Design review of the part built by this model. Coordinates are the model's own, in mm. A direction names the side the tool comes from. Coordinates: 2 decimals unless noted, no trailing zeros. Order: outer loops, then holes, each group sorted by start corner. A loop starts at its lowest first (then second) coordinate and runs counter-clockwise, first axis right, second up. Notation, with made-up numbers: M 54.25,-2.75 L 66.25,-2.75 A32 cw 66.25,28.25 Z; hole C 16.5,52 d10. An arc over 180 degrees is marked long. Answer in a Markdown table with one row per item.
from build123d import *

# Parameters (mm, degrees)
F0_R     = 76.2
F1_DEPTH = 6.35
F3_DEPTH = 3.81


with BuildPart() as f1:
    # F0 (on Top) → F1 (new body)
    with BuildSketch(Plane.XY):
        Circle(F0_R)
    extrude(amount=F1_DEPTH)

    # F2 (on face) → F3 (cut)
    with BuildSketch(Plane.XY.offset(6.35)):
        with BuildLine():
            Line((0, 76.2), (-1.27, 76.2))
            Line((-1.27, 76.2), (-1.27, 76.1894159316))
            ThreePointArc((-1.27, 76.1894159316), (-0.6350220513, 76.197353937), (0, 76.2))
        make_face()
        with BuildLine():
            Line((1.27, 76.2), (0, 76.2))
            ThreePointArc((0, 76.2), (0.6350220513, 76.197353937), (1.27, 76.1894159316))
            Line((1.27, 76.1894159316), (1.27, 76.2))
        make_face()
        with BuildLine():
            ThreePointArc((0, -76.2), (-0.6350220513, -76.197353937), (-1.27, -76.1894159316))
            Line((-1.27, -76.1894159316), (-1.27, -76.2))
            Line((-1.27, -76.2), (0, -76.2))
        make_face()
        with BuildLine():
            Line((1.27, -76.2), (1.27, -76.1894159316))
            ThreePointArc((1.27, -76.1894159316), (0.6350220513, -76.197353937), (0, -76.2))
            Line((0, -76.2), (1.27, -76.2))
        make_face()
        with BuildLine():
            ThreePointArc((1.27, 76.1894159316), (0.6350220513, 76.197353937), (0, 76.2))
            ThreePointArc((0, 76.2), (-0.6350220513, 76.197353937), (-1.27, 76.1894159316))
            Line((-1.27, 76.1894159316), (-1.27, -76.1894159316))
            ThreePointArc((-1.27, -76.1894159316), (-0.6350220513, -76.197353937), (0, -76.2))
            ThreePointArc((0, -76.2), (0.6350220513, -76.197353937), (1.27, -76.1894159316))
            Line((1.27, -76.1894159316), (1.27, 76.1894159316))
        make_face()
    extrude(amount=-F3_DEPTH, mode=Mode.SUBTRACT)


solid = f1.part
(1) Add section A-A, the plane z = 4.25. Give the boundary of the cut face in (x, y).
Return value:
| item | result |
|---|---|
| outline | M -1.27,-76.19 L -1.27,76.19 A76.2 ccw Z; M 1.27,-76.19 A76.2 ccw 1.27,76.19 Z |
(2) Add section B-B, the plane y = -13. Give the boundary of the cut face in (x, z).
Return value:
| item | result |
|---|---|
| outline | M -75.08,0 L 75.08,0 L 75.08,6.35 L 1.27,6.35 L 1.27,2.54 L -1.27,2.54 L -1.27,6.35 L -75.08,6.35 Z |
(3) Add section D-D, the plane y = -39.5. Give the boundary of the cut face in (x, z).
Return value:
| item | result |
|---|---|
| outline | M -65.16,0 L 65.16,0 L 65.16,6.35 L 1.27,6.35 L 1.27,2.54 L -1.27,2.54 L -1.27,6.35 L -65.16,6.35 Z |
(4) For line 1 along X through (y, z) = (-1, 6.25); line 2 along X through (y, z) = (23, 5.25); line 3 along Y through (x, z) = (-56, 2.25), list the stretches that pass through material, from the lowest coordinate up. Write a range as from..to.
Return value:
| item | result |
|---|---|
| line 1 | x = -76.19..-1.27, 1.27..76.19 |
| line 2 | x = -72.65..-1.27, 1.27..72.65 |
| line 3 | y = -51.68..51.68 |
(5) For faces 4 (the flat face through (30, 1, 6.35)), 5 (the flat face through (-1.27, 1, 4)), list the 3-axis set-ups (+Z, -Z, +X, -X, +Y, -Y) from which the entire face can be reached by the end or side of a thin tool; tool diameter is ignored.
Return value:
| item | result |
|---|---|
| face 4 | +Z, +X, -X, +Y, -Y |
| face 5 | +Z, +Y, -Y |
(6) Draft analysis for pull direction X (two halves, no side actions). For faces 1 (the cylindrical face through (-60.47, -46.367, 3.131)), 2 (the flat face through (-31, 1, 6.35)), 3 (the flat face through (1.27, -1, 4)), state which applies: pulls with the +X half, pulls with the -X half, needs draft (parallel to the pull), parting line crosses it, or undercut.
Return value:
| item | result |
|---|---|
| face 1 | parting line crosses it |
| face 2 | needs draft |
| face 3 | undercut |
(7) Insertion check: pin 1 Ø1.5 at (y, z) = (38, 2.5) entering from +X; pin 2 Ø2 at (x, z) = (49.5, 5) entering from +Y; pin 3 Ø1 at (y, z) = (-26.5, 1.5) entering from -X. Each pin has a flat end and moves straight along its axis. Give the tip position at first contact, or say it passes through.
Return value:
| item | result |
|---|---|
| pin 1 | stops at x = 66.47 |
| pin 2 | stops at y = 58.77 |
| pin 3 | stops at x = -71.63 |
(8) Add section C-C, the plane x = 21.5. Give the boundary of the cut face in (y, z).
Return value:
| item | result |
|---|---|
| outline | M -73.1,0 L 73.1,0 L 73.1,6.35 L -73.1,6.35 Z |
